```python
from build123d import *

# Parameters (mm, degrees)
F0_W      = 100
F0_H      = 100
F1_DEPTH  = 50
F2_T      = -3
F3_R      = 5.5
F4_DEPTH  = 50
F5_R      = 20
F5_R_2    = 17.5
F6_DEPTH  = 25
F7_DEPTH  = 3
F8_W      = 10
F8_H      = 20
F9_DEPTH  = 15
F10_R     = 5.3726460022
F11_DEPTH = 100
F12_R     = 8
F13_R     = 7
F13_R_2   = 5.5
F14_DEPTH = 3
F15_W     = 100
F15_H     = 50
F16_DEPTH = 3
F18_DEPTH = 50
F20_W     = 100
F20_H     = 50
F20_W_2   = 94
F20_H_2   = 44
F21_DEPTH = 50
F22_R     = 12.5
F23_DEPTH = 53
F24_W     = 100
F24_H     = 50
F25_DEPTH = 3
F26_R     = 14
F26_R_2   = 12.5
F27_DEPTH = 25
F28_DEPTH = 3
F30_DEPTH = 44


with BuildPart() as f1:
    # F0 (on Top) → F1 (new body)
    with BuildSketch(Plane.XY):
        Rectangle(F0_W, F0_H)
    extrude(amount=F1_DEPTH)

    # F2
    f2_openings = [f1.faces().sort_by_distance(p)[0] for p in [
        (0, 50, 25),
    ]]
    offset(amount=F2_T, openings=f2_openings)

    # F3 (on face) → F4 (cut, through all)
    with BuildSketch(Plane.XY.offset(50)):
        Circle(F3_R)
    extrude(amount=-F4_DEPTH, mode=Mode.SUBTRACT)

    # F5 (on face) → F6 (join)
    with BuildSketch(Plane.XZ.offset(50)):
        with Locations((0, 25)):
            Circle(F5_R)
        with Locations((0, 25)):
            Circle(F5_R_2, mode=Mode.SUBTRACT)
    extrude(amount=F6_DEPTH)

    # F5 (on face) → F7 (cut, through all)
    with BuildSketch(Plane.XZ.offset(50)):
        with Locations((0, 25)):
            Circle(F5_R_2)
    extrude(amount=-F7_DEPTH, mode=Mode.SUBTRACT)

    # F8 (on face) → F9 (join)
    with BuildSketch(Plane(origin=(0, 0, 0), x_dir=(1, 0, 0), z_dir=(0, 0, -1))):
        with Locations((45, -40)):
            Rectangle(F8_W, F8_H)
        with Locations((-45, -40)):
            Rectangle(F8_W, F8_H)
        with Locations((-45, 40)):
            Rectangle(F8_W, F8_H)
        with Locations((45, 40)):
            Rectangle(F8_W, F8_H)
    extrude(amount=F9_DEPTH)

    # F10 (on face) → F11 (cut, through all)
    with BuildSketch(Plane.YZ.offset(50)):
        with Locations((40, -7)):
            Circle(F10_R)
        with Locations((-40, -7)):
            Circle(F10_R)
    extrude(amount=-F11_DEPTH, mode=Mode.SUBTRACT)

    # F12
    f12_edges = [f1.edges().sort_by_distance(p)[0] for p in [
        (45, 30, -15),
        (45, 50, -15),
        (-45, 50, -15),
        (-45, 30, -15),
        (45, -50, -15),
        (45, -30, -15),
        (-45, -50, -15),
        (-45, -30, -15),
    ]]
    fillet(f12_edges, radius=F12_R)

    # F13 (on face) → F14 (join)
    with BuildSketch(Plane.XY.offset(3)):
        Circle(F13_R)
        Circle(F13_R_2, mode=Mode.SUBTRACT)
    extrude(amount=F14_DEPTH)

    # F15 (on face) → F16 (join)
    with BuildSketch(Plane(origin=(0, 50, 0), x_dir=(-1, 0, 0), z_dir=(0, 1, 0))):
        with Locations((0, 25)):
            Rectangle(F15_W, F15_H)
    extrude(amount=F16_DEPTH)

    # F17 (on Top) → F18 (join, through all)
    with BuildSketch(Plane.XY):
        Polygon((-50, 53), (50, 53), (50, 79.7949192431), align=None)
    extrude(amount=F18_DEPTH)

    # F20 (on face) → F21 (join)
    with BuildSketch(Plane(origin=(0, 53, 0), x_dir=(-1, 0, 0), z_dir=(0, 1, 0))):
        with Locations((0, 25)):
            Rectangle(F20_W, F20_H)
        with Locations((0, 25)):
            Rectangle(F20_W_2, F20_H_2, mode=Mode.SUBTRACT)
    extrude(amount=F21_DEPTH)

    # F22 (on face) → F23 (cut, through all)
    with BuildSketch(Plane(origin=(0, 103, 0), x_dir=(-1, 0, 0), z_dir=(0, 1, 0))):
        with Locations((30, 25)):
            Circle(F22_R)
    extrude(amount=-F23_DEPTH, mode=Mode.SUBTRACT)

    # F24 (on face) → F25 (join)
    with BuildSketch(Plane(origin=(0, 103, 0), x_dir=(-1, 0, 0), z_dir=(0, 1, 0))):
        with Locations((0, 25)):
            Rectangle(F24_W, F24_H)
    extrude(amount=F25_DEPTH)

    # F26 (on face) → F27 (join)
    with BuildSketch(Plane(origin=(0, 106, 0), x_dir=(-1, 0, 0), z_dir=(0, 1, 0))):
        with Locations((-31.1048589647, 25)):
            Circle(F26_R)
        with Locations((-31.1048589647, 25)):
            Circle(F26_R_2, mode=Mode.SUBTRACT)
    extrude(amount=F27_DEPTH)

    # F28 (cut, through all): a face of the model
    f28_faces = [f1.faces().sort_by_distance(p)[0] for p in [
        (31.1048589647, 106, 25),
    ]]
    extrude(f28_faces, amount=-F28_DEPTH, mode=Mode.SUBTRACT)

    # F29 (on face) → F30 (join, through all)
    with BuildSketch(Plane.XY.offset(3)):
        Polygon((-34.5411077142, 28.4994188696), (-41.7947806418, 50), (-47, 50), (-47, 28.4994188696), align=None)
    extrude(amount=F30_DEPTH)


solid = f1.part
```
Geometry check sheet. Reference: the model listing, model coordinates, mm. A direction names the side the tool comes from. Coordinates: 2 decimals unless noted, no trailing zeros. Order: outer loops, then holes, each group sorted by start corner. A loop starts at its lowest first (then second) coordinate and runs counter-clockwise, first axis right, second up. Notation, with made-up numbers: (-5, 63) - (31, 63) arc R19 ccw to (31, 89) - close; hole circle Ø3 at (25.5, 41.5). An arc over 180 degrees is marked (long way). Answer in a Markdown table with one row per item. Add a question column.
1. Material ranges on L1, parallel to Z at x = 46.75, y = -40; L2, parallel to Z at x = 19.5, y = 22; L3, parallel to Z at x = 47.25, y = 40, recorded low to high. Write a range as [from, to].
2. Section check C-C (z = -9.5). Give the number of separate pieces and of enclosed holes in the cut face, plus the area to 3 significant figures.
3. Access from +Z, -Z, +X, -X, +Y, -Y to the whole of each face (thin tool, end or side, straight path). Record for faces 1 (the face through (34.14, 118.325, 11.333)), 2 (the face through (-40, 45, -4)), 3 (the face through (45.07, -32.281, -12.594)), 4 (the face through (10, 2, 47)), 5 (the face through (45.07, 47.719, -12.594)).
4. Gauge pin test, flat ends, axial feed: pin 1 Ø12 at (y, z) = (40, -6) entering from +X; pin 2 Ø17.5 at (x, y) = (0, 0) entering from -Z; pin 3 Ø2 at (x, z) = (44, -2.5) entering from +Y; pin 4 Ø2 at (x, z) = (-30.5, 38.5) entering from -Y. Record the tip position at first contact, or that the pin passes through.
5. Section check B-B (y = 24.5). Enter the section's corners in (x, z), plus the area to 3 significant figures.
6. Draft check along Y on faces 6 (the face through (-2.28, -60.8, 42.35)), 7 (the face through (45.07, -47.719, -12.594)), 8 (the face through (-47, -10, 25)), 9 (the face through (-44.93, 47.719, -12.594)). Enter one of: +Y half, -Y half, draft (parallel to the pull), parting line (faces both ways), or undercut.
7. Section check A-A (y = 0). Enter the section's corners in (x, z).
Data:
| question | item | result |
|---|---|---|
| 1 | L1 | z = [-15, -12.37], [-1.63, 3], [47, 50] |
| 1 | L2 | z = [0, 3], [47, 50] |
| 1 | L3 | z = [-15, -12.37], [-1.63, 50] |
| 2 | separate pieces | 8 |
| 2 | enclosed holes | 0 |
| 2 | area | 388 mm² |
| 3 | face 1 | +Y |
| 3 | face 2 | -Z, +Y, -Y |
| 3 | face 3 | -Z, +X, -X |
| 3 | face 4 | none |
| 3 | face 5 | -Z, +X, -X, +Y |
| 4 | pin 1 | stops at x = 50 |
| 4 | pin 2 | stops at z = 0 |
| 4 | pin 3 | stops at y = 50 |
| 4 | pin 4 | stops at y = -50 |
| 5 | outline | (-50, 0) - (50, 0) - (50, 50) - (-50, 50) - close; hole (-47, 3) - (47, 3) - (47, 47) - (-47, 47) - close |
| 5 | area | 864 mm² |
| 6 | face 6 | draft |
| 6 | face 7 | -Y half |
| 6 | face 8 | undercut |
| 6 | face 9 | +Y half |
| 7 | outline | (-50, 0) - (-5.5, 0) - (-5.5, 6) - (-7, 6) - (-7, 3) - (-47, 3) - (-47, 47) - (-5.5, 47) - (-5.5, 50) - (-50, 50) - close; (5.5, 0) - (50, 0) - (50, 50) - (5.5, 50) - (5.5, 47) - (47, 47) - (47, 3) - (7, 3) - (7, 6) - (5.5, 6) - close |
